For this review, take the finished solid that the model builds, in its own axes (mm). Give positions to 0.01 mm unless a question says otherwise; leave off trailing zeros. Order: outer loops, then holes, each group sorted by start corner. A loop starts at its lowest first (then second) coordinate and runs counter-clockwise, first axis right, second up. Notation, with made-up numbers: M 20,13.5 L 31,13.5 A23 cw 31,37.5 Z; hole C 77.5,25 d11. An arc over 180 degrees is marked long. Use CSV: the item, a comma, the result in double quotes. Start each with the question number.
(1) Wall thickness on L1, parallel to Y at x = -12.5, z = 3.5; L2, parallel to X at y = 31, z = 5.25; L3, parallel to Y at x = -1.5, z = 8.5: over which ranges is each line inside the solid? List them lowest first. Write a range as from..to.
(2) Consider section A-A (x = 18.5). Write out the cut boundary in (y, z).
(3) Consider section C-C (z = 6.25). Write out the cut boundary in (x, y), and give its area (3 significant figures).
(4) Consider section B-B (y = 0). Write out the cut boundary in (x, z).
(5) Consider section D-D (y = 28). Write out the cut boundary in (x, z).
```python
from build123d import *

# Parameters (mm, degrees)
F0_R     = 1.75
F0_R_2   = 12
F0_R_3   = 2.75
F1_DEPTH = 9


with BuildPart() as f1:
    # F0 (on Top) → F1 (new body)
    with BuildSketch(Plane.XY):
        with BuildLine():
            Line((19.5, 39), (-19.5, 39))
            ThreePointArc((-19.5, 39), (-23.035534, 37.535534), (-24.5, 34))
            Line((-24.5, 34), (-24.5, -10))
            ThreePointArc((-24.5, -10), (-23.035534, -13.535534), (-19.5, -15))
            Line((-19.5, -15), (19.5, -15))
            ThreePointArc((19.5, -15), (23.035534, -13.535534), (24.5, -10))
            Line((24.5, -10), (24.5, 34))
            ThreePointArc((24.5, 34), (23.035534, 37.535534), (19.5, 39))
        make_face()
        with Locations((-18.5, 5)):
            Circle(F0_R, mode=Mode.SUBTRACT)
        Circle(F0_R_2, mode=Mode.SUBTRACT)
        with Locations((18.5, 5)):
            Circle(F0_R, mode=Mode.SUBTRACT)
        with Locations((-12.5, 29)):
            Circle(F0_R_3, mode=Mode.SUBTRACT)
        with Locations((12.5, 29)):
            Circle(F0_R_3, mode=Mode.SUBTRACT)
    extrude(amount=F1_DEPTH)


solid = f1.part
```
Check result:
1,L1,"y = -15..26.25, 31.75..39"
1,L2,"x = -24.5..-14.39, -10.61..10.61, 14.39..24.5"
1,L3,"y = -15..-11.91, 11.91..39"
2,outline,"M -15,0 L 3.25,0 L 3.25,9 L -15,9 Z; M 6.75,0 L 39,0 L 39,9 L 6.75,9 Z"
3,outline,"M -24.5,-10 A5 ccw -19.5,-15 L 19.5,-15 A5 ccw 24.5,-10 L 24.5,34 A5 ccw 19.5,39 L -19.5,39 A5 ccw -24.5,34 Z; hole C -18.5,5 d3.5; hole C -12.5,29 d5.5; hole C 0,0 d24; hole C 12.5,29 d5.5; hole C 18.5,5 d3.5"
3,area,"2,110 mm^2"
4,outline,"M -24.5,0 L -12,0 L -12,9 L -24.5,9 Z; M 12,0 L 24.5,0 L 24.5,9 L 12,9 Z"
5,outline,"M -24.5,0 L -15.06,0 L -15.06,9 L -24.5,9 Z; M -9.94,0 L 9.94,0 L 9.94,9 L -9.94,9 Z; M 15.06,0 L 24.5,0 L 24.5,9 L 15.06,9 Z"
